```python
from build123d import *

# Parameters (mm, degrees)
BOSS_EXTRUDE2_DEPTH  = 8
ROD_POCKET_DEPTH     = 6
POCKET_FILLETS_R     = 1
PROFILE_FILLETS_R    = 2
INSERT_CHAM_SIZE     = 0.5
SKETCH6_R            = 2.875
COUNTERSINK_DEPTH    = 2.6
SKETCH7_R            = 1.575
THROUGH_HOLE_DEPTH   = 47.262360557
DEBURS_SIZE          = 0.2
OUTSIDE_CHAMFER_SIZE = 0.75


with BuildPart() as part:
    # Sketch1 → Boss-Extrude2 (new body)
    with BuildSketch(Plane.XY):
        with BuildLine():
            Line((-7.505553499, -38.45), (-4.486437749, 0.349107895))
            ThreePointArc((-4.486437749, 0.349107895), (0, 4.5), (4.486437749, 0.349107895))
            Line((4.486437749, 0.349107895), (7.505553499, -38.45))
            Line((7.505553499, -38.45), (3.75277675, -44.95))
            Line((3.75277675, -44.95), (-3.75277675, -44.95))
            Line((-3.75277675, -44.95), (-7.505553499, -38.45))
        make_face()
    extrude(amount=BOSS_EXTRUDE2_DEPTH)

    # Sketch5 → Rod Pocket (cut)
    with BuildSketch(Plane.XY.offset(8)):
        Polygon((5.183091381, -27.938688806), (2.59154569, -23.45), (-2.59154569, -23.45), (-5.183091381, -27.938688806), (-5.973996897, -38.102733849), (-2.886751346, -43.45), (2.886751346, -43.45), (5.973996897, -38.102733849), align=None)
    extrude(amount=-ROD_POCKET_DEPTH, mode=Mode.SUBTRACT)

    # Pocket Fillets
    pocket_fillets_edges = [part.edges().sort_by_distance(p)[0] for p in [
        (2.59154569, -23.45, 5),
        (-2.59154569, -23.45, 5),
        (-5.183091381, -27.938688806, 5),
        (-5.973996897, -38.102733849, 5),
        (-2.886751346, -43.45, 5),
        (2.886751346, -43.45, 5),
        (5.973996897, -38.102733849, 5),
        (5.183091381, -27.938688806, 5),
    ]]
    fillet(pocket_fillets_edges, radius=POCKET_FILLETS_R)

    # Profile Fillets
    profile_fillets_edges = [part.edges().sort_by_distance(p)[0] for p in [
        (7.505553499, -38.45, 4),
        (3.75277675, -44.95, 4),
        (-3.75277675, -44.95, 4),
        (-7.505553499, -38.45, 4),
    ]]
    fillet(profile_fillets_edges, radius=PROFILE_FILLETS_R)

    # Insert Cham
    insert_cham_edges = [part.edges().sort_by_distance(p)[0] for p in [
        (-5.575313572, -32.979194827, 8),
        (-3.974970938, -25.846162818, 8),
        (-4.497205523, -40.660611541, 8),
        (0, -43.45, 8),
        (4.497205523, -40.660611541, 8),
        (5.575313572, -32.979194827, 8),
        (3.974970938, -25.846162818, 8),
        (0, -23.45, 8),
        (-5.158846312, -27.946205375, 8),
        (-5.928204033, -38.092350745, 8),
        (-2.809401077, -43.316025404, 8),
        (2.809401077, -43.316025404, 8),
        (5.928204033, -38.092350745, 8),
        (5.158846312, -27.946205375, 8),
        (2.514195421, -23.583974596, 8),
        (-2.514195421, -23.583974596, 8),
    ]]
    chamfer(insert_cham_edges, length=INSERT_CHAM_SIZE)

    # Sketch6 → Countersink (cut)
    with BuildSketch(Plane(origin=(0, 0, 0), x_dir=(-1, 0, 0), z_dir=(0, 0, -1))):
        Circle(SKETCH6_R)
    extrude(amount=-COUNTERSINK_DEPTH, mode=Mode.SUBTRACT)

    # Sketch7 → Through Hole (cut, through all)
    with BuildSketch(Plane.XY):
        with Locations(Location((0, 0, 0), (0, 0, 180))):
            Circle(SKETCH7_R)
    extrude(amount=THROUGH_HOLE_DEPTH, mode=Mode.SUBTRACT)

    # Deburs
    deburs_edges = [part.edges().sort_by_distance(p)[0] for p in [
        (5.762827928, -41.468489233, 8),
        (-5.762827928, -41.468489233, 8),
        (0, -44.95, 8),
        (-3.598076211, -44.682050808, 8),
        (3.598076211, -44.682050808, 8),
        (-7.41396777, -38.429233792, 8),
        (7.41396777, -38.429233792, 8),
        (2.875, 0, 0),
        (1.575, 0, 2.6),
        (1.575, 0, 8),
        (0, 4.5, 8),
        (-5.971944056, -18.741355754, 8),
        (5.971944056, -18.741355754, 8),
    ]]
    chamfer(deburs_edges, length=DEBURS_SIZE)

    # Outside Chamfer
    outside_chamfer_edges = [part.edges().sort_by_distance(p)[0] for p in [
        (-3.598076211, -44.682050808, 0),
        (3.598076211, -44.682050808, 0),
        (-7.41396777, -38.429233792, 0),
        (7.41396777, -38.429233792, 0),
        (-5.971944056, -18.741355754, 0),
        (0, 4.5, 0),
        (5.971944056, -18.741355754, 0),
        (5.762827928, -41.468489233, 0),
        (0, -44.95, 0),
        (-5.762827928, -41.468489233, 0),
    ]]
    chamfer(outside_chamfer_edges, length=OUTSIDE_CHAMFER_SIZE)


solid = part.part
```
For this review, take the finished solid that the model builds, in its own axes (mm). A direction names the side the tool comes from. Coordinates: 2 decimals unless noted, no trailing zeros. Loops run counter-clockwise (first coordinate to the right, second up) from the corner with the lowest first, then second, coordinate; pieces in that order, holes last.
1. Add section B-B, the plane z = 5. Give the boundary of the cut face in (x, y) (3 decimals).
2. Mouldability with a two-part tool opening along X and no side actions: class faces 3 (the flat face through (0, -44.95, 4)), 4 (the flat face through (-2, 0, 2.6)), 5 (the flat face through (-4.173, -25.696, 7.746)), 6 (the cylindrical face through (-3.611, -44.675, 4.324)) as +X half, -X half, draft (parallel to the pull), parting line (faces both ways), or undercut.
3. For line 1 (Y direction, x = 0, z = 2.15) (3 decimals); line 2 (Y direction, x = 0, z = 1.5) (3 decimals); line 3 (Y direction, x = 0, z = 4) (3 decimals), list the stretches that pass through material, from the lowest coordinate up.
4. Insertion check: P1, Ø3, axis at x = 0, y = 0, coming from the +Z side; P2, Ø4.5, axis at x = 0.5, y = 0, coming from the -Z side; P3, Ø1, axis at x = -2, z = 6.5, coming from the +Y side; P4, Ø2, axis at y = -10.5, z = 1, coming from the -X side. Each pin has a flat end and moves straight along its axis. Give the tip position at first contact, or say it passes through.
5. Add section C-C, the plane z = 1.5. Give the boundary of the cut face in (x, y) (3 decimals), then the cut area to 3 significant figures.
6. Add section D-D, the plane y = -31.5. Give the boundary of the cut face in (x, z).
7. For faces 1 (the conical face through (-2.6, -23.4, 7.7)), 2 (the flat face through (0, -25, 0)), list the 3-axis set-ups (+Z, -Z, +X, -X, +Y, -Y) from which the entire face can be reached by the end or side of a thin tool; tool diameter is ignored.
8. Add section A-A, the plane x = 0. Give the boundary of the cut face in (y, z) (3 decimals), then the cut area to 3 significant figures.
Result:
1. outline: (-7.457, -37.832) arc R2 ccw to (-7.196, -38.987) - (-4.33, -43.95) arc R2 ccw to (-2.598, -44.95) - (2.598, -44.95) arc R2 ccw to (4.33, -43.95) - (7.196, -38.987) arc R2 ccw to (7.457, -37.832) - (4.486, 0.349) arc R4.5 ccw to (-4.486, 0.349) - close; hole (-5.95, -37.794) arc R1 ccw to (-5.819, -38.371) - (-3.175, -42.95) arc R1 ccw to (-2.309, -43.45) - (2.309, -43.45) arc R1 ccw to (3.175, -42.95) - (5.819, -38.371) arc R1 ccw to (5.95, -37.794) - (5.201, -28.165) arc R1 ccw to (5.07, -27.742) - (2.88, -23.95) arc R1 ccw to (2.014, -23.45) - (-2.014, -23.45) arc R1 ccw to (-2.88, -23.95) - (-5.07, -27.742) arc R1 ccw to (-5.201, -28.165) - close; hole circle Ø3.15 at (0, 0)
2. face 3: draft
2. face 4: undercut
2. face 5: undercut
2. face 6: -X half
3. line 1: y = -44.95 to -43.45, -23.45 to -2.875, 2.875 to 4.5
3. line 2: y = -44.95 to -2.875, 2.875 to 4.5
3. line 3: y = -44.95 to -43.45, -23.45 to -1.575, 1.575 to 4.5
4. P1: passes through
4. P2: stops at z = 2.6
4. P3: stops at y = 4.24
4. P4: stops at x = -5.41
5. outline: (-7.457, -37.832) arc R2 ccw to (-7.196, -38.987) - (-4.33, -43.95) arc R2 ccw to (-2.598, -44.95) - (2.598, -44.95) arc R2 ccw to (4.33, -43.95) - (7.196, -38.987) arc R2 ccw to (7.457, -37.832) - (4.486, 0.349) arc R4.5 ccw to (-4.486, 0.349) - close; hole circle Ø5.75 at (0, 0)
5. area: 541 mm2
6. outline: (-6.96, 0.75) - (-6.21, 0) - (6.21, 0) - (6.96, 0.75) - (6.96, 7.8) - (6.76, 8) - (5.96, 8) - (5.46, 7.5) - (5.46, 2) - (-5.46, 2) - (-5.46, 7.5) - (-5.96, 8) - (-6.76, 8) - (-6.96, 7.8) - close
7. face 1: +Z
7. face 2: -Z, +X, -X, +Y, -Y
8. outline: (-44.95, 0.75) - (-44.2, 0) - (-3.075, 0) - (-2.875, 0.2) - (-2.875, 2.6) - (-1.775, 2.6) - (-1.575, 2.8) - (-1.575, 7.8) - (-1.775, 8) - (-22.95, 8) - (-23.45, 7.5) - (-23.45, 2) - (-43.45, 2) - (-43.45, 7.5) - (-43.95, 8) - (-44.75, 8) - (-44.95, 7.8) - close; (1.575, 2.8) - (1.775, 2.6) - (2.875, 2.6) - (2.875, 0.2) - (3.075, 0) - (3.75, 0) - (4.5, 0.75) - (4.5, 7.8) - (4.3, 8) - (1.775, 8) - (1.575, 7.8) - close
8. area: 243 mm2
